Geometry: final body of the model. Coordinates: model frame, mm. A direction names the side the tool comes from. Coordinates: 2 decimals unless noted, no trailing zeros. Write each loop counter-clockwise with the first axis right and the second up, starting at its lowest first coordinate (ties: lowest second). Pieces come first, ordered by that corner, then holes.
Autodesk Inventor part; units mm, degrees
ref_plane "YZ Plane" through (0, 0, 0) normal (1, 0, 0) x (0, 1, 0)
ref_plane "XZ Plane" through (0, 0, 0) normal (0, 1, 0) x (-1, 0, 0)
ref_plane "XY Plane" through (0, 0, 0) normal (0, 0, 1) x (1, 0, 0)
sketch "スケッチ1" plane through (0, 0, 0) normal (1, 0, 0) x (0, 1, 0)
  circle A0 centre (0, 0) radius 65
  circle A1 centre (0, 0) radius 52.5
  dimension "d0" = 130
  dimension "d1" = 105
extrude "押し出し1" add sketch "スケッチ1" along normal blind 13
fillet "フィレット1" radius 1 4 edges at (13, -65, 0) (0, -65, 0) (13, -52.5, 0) (0, -52.5, 0)
sketch "スケッチ2" plane through (13, 0, 0) normal (1, 0, 0) x (0, 0, -1)
  circle A0 centre (0, 0) radius 55.1
  circle A1 centre (0, 0) radius 52.5
  circle A2 centre (0, 0) radius 62.7
  circle A3 centre (0, 0) radius 65
  dimension "d5" = 2.6
  dimension "d6" = 2.3
extrude "押し出し2" cut sketch "スケッチ2" against normal blind 0.7 contours A2
sketch "スケッチ3" plane through (0, 0, 0) normal (-1, 0, 0) x (0, 0, 1)
  circle A0 centre (0, 0) radius 55.1
  circle A1 centre (0, 0) radius 62.7
extrude "押し出し3" cut sketch "スケッチ3" against normal blind 0.7
properties part number "Bearing_Large"
Item 1: Section C-C, the plane x = 4.5. Output: boundary loops of the cut face in (y, z), plus the area to 3 significant figures.
Derived:
outline: circle Ø130 at (0, 0); hole circle Ø105 at (0, 0)
area: 4,610 mm2
Item 2: Set-up query: faces 1 (the cylindrical face through (0.345, 16.551, 52.556)), 2 (the cylindrical face through (12.65, -61.21, 13.59)), 3 (the flat face through (0, -8.4, 53.3)). Return all of +Z, -Z, +X, -X, +Y, -Y with unobstructed straight access to the full face (end or side cutting, diameter ignored); none if empty.
Derived:
face 1: -X
face 2: +X
face 3: +Z, -Z, -X, +Y, -Y
Item 3: Material intervals for probe 1 along Z at (x, y) = (3.5, 0); probe 2 along Y at (x, z) = (4.5, -20.5); probe 3 along Y at (x, z) = (6.75, 21), sorted ascending.
Derived:
probe 1: z = -65 to -52.5, 52.5 to 65
probe 2: y = -61.68 to -48.33, 48.33 to 61.68
probe 3: y = -61.51 to -48.12, 48.12 to 61.51
Item 4: Pin query (flat end, axial travel): pin 1 (5 mm diameter, centred on x = 9, z = 28.5, fed in from -Y); pin 2 (2 mm diameter, centred on x = 4.5, y = -3.5, fed in from -Z); pin 3 (4 mm diameter, centred on x = 7, z = -42.5, fed in from +Y); pin 4 (3 mm diameter, centred on y = -37.5, z = -49.5, fed in from +X). Return the tip coordinate at first contact, or that it passes through.
Derived:
pin 1: stops at y = -59.57
pin 2: stops at z = -64.95
pin 3: stops at y = 50.84
pin 4: stops at x = 13
Item 5: Pull-direction query (Z, two-part tool) for faces 4 (the flat face through (12.3, -55.4, 0.3)), 5 (the cylindrical face through (6.42, 62, -19.52)), 6 (the flat face through (13, -8.4, 53.3)); classes: released by +Z, released by -Z, zero draft, split by the parting line, or undercut.
Derived:
face 4: undercut
face 5: split by the parting line
face 6: zero draft
